from build123d import *

# Parameters (mm, degrees)
F1_DEPTH = 22
F4_DEPTH = 19
F5_R     = 2.5
F6_DEPTH = 5
F7_R     = 4.5
F8_DEPTH = 8


with BuildPart() as f1:
    # F0 (on Top) → F1 (new body)
    with BuildSketch(Plane.XY):
        with BuildLine():
            ThreePointArc((-32.5, 0), (0, 25), (32.5, 0))
            Line((32.5, 0), (49.369318, 0))
            Line((49.369318, 0), (49.369318, 2.5))
            Line((49.369318, 2.5), (34.369318, 2.5))
            ThreePointArc((34.369318, 2.5), (0, 27.5), (-34.369318, 2.5))
            Line((-34.369318, 2.5), (-49.369318, 2.5))
            Line((-49.369318, 2.5), (-49.369318, 0))
            Line((-49.369318, 0), (-32.5, 0))
        make_face()
        with BuildLine():
            Line((49.369318, 0), (32.5, 0))
            ThreePointArc((32.5, 0), (0, -25), (-32.5, 0))
            Line((-32.5, 0), (-49.369318, 0))
            Line((-49.369318, 0), (-49.369318, -2.5))
            Line((-49.369318, -2.5), (-34.369318, -2.5))
            ThreePointArc((-34.369318, -2.5), (0, -27.5), (34.369318, -2.5))
            Line((34.369318, -2.5), (49.369318, -2.5))
            Line((49.369318, -2.5), (49.369318, 0))
        make_face()
    extrude(amount=F1_DEPTH)

    # F3 (on offset) → F4 (join)
    with BuildSketch(Plane.XZ.offset(25)):
        Polygon((6, 11), (2.932883, 16), (-2.932883, 16), (-6, 11), (-2.932883, 6), (2.932883, 6), align=None)
    extrude(amount=F4_DEPTH)

    # F5 (on face) → F6 (cut, through all)
    with BuildSketch(Plane.XZ.offset(2.5)):
        with Locations((41.5, 11)):
            Circle(F5_R)
        with Locations((-41.5, 11)):
            Circle(F5_R)
    extrude(amount=-F6_DEPTH, mode=Mode.SUBTRACT)

    # F7 (on face) → F8 (cut)
    with BuildSketch(Plane.XZ.offset(44)):
        with Locations((0, 11)):
            Circle(F7_R)
    extrude(amount=-F8_DEPTH, mode=Mode.SUBTRACT)


solid = f1.part
Geometry check sheet. Reference: the model listing, model coordinates, mm. A direction names the side the tool comes from. Round coordinates to 2 decimals unless told otherwise and drop trailing zeros. Order: outer loops, then holes, each group sorted by start corner. A loop starts at its lowest first (then second) coordinate and runs counter-clockwise, first axis right, second up. Notation, with made-up numbers: M 83,86.25 L 137,86.25 A18 ccw 137,94.25 Z; hole C -20.75,65 d9. An arc over 180 degrees is marked long. Answer in a Markdown table with one row per item. Add a question column.
Item 1: Draft check along X on faces 5 (the face through (49.369, 0, 11)), 6 (the face through (0, -36, 11)), 7 (the face through (-49.369, 0, 11)). Enter one of: released by +X, released by -X, zero draft, split by the parting line, or undercut.
Item 2: Sectioned sample at A-A, the plane x = 0. Enter the section's corners in (y, z), plus the area to 3 significant figures.
Item 3: Material ranges on L1, parallel to Z at x = 0, y = -39.75; L2, parallel to Z at x = 41.5, y = 0.05; L3, parallel to Y at x = 44.5, z = 16, recorded low to high. Write a range as [from, to].
Item 4: Sectioned sample at D-D, the plane x = -41.5. Enter the section's corners in (y, z).
Item 5: Sectioned sample at B-B, the plane z = 19.25. Enter the section's corners in (x, y) (3 decimals).
Item 6: Sectioned sample at C-C, the plane y = 3.5. Enter the section's corners in (x, z), plus the area to 3 significant figures.
Item 7: Set-up check for faces 1 (the face through (42, 2.5, 8)), 2 (the face through (4.49, -35.38, 13.46)), 3 (the face through (4.44, -35.38, 8.46)), 4 (the face through (-42, -2.5, 8)): record each of +Z, -Z, +X, -X, +Y, -Y from which the full face is reachable in a straight line by a thin tool's end or side.
Item 8: Depth check by flat-ended pin: pin 1 Ø8 at (y, z) = (-27.5, 11) entering from +X; pin 2 Ø4 at (y, z) = (-18, 5) entering from +X; pin 3 Ø12 at (y, z) = (10.5, 8) entering from +X; pin 4 Ø10 at (x, y) = (-12, 12) entering from +Z. Enter the tip coordinate at first touch or a pass-through.
Filled in:
| question | item | result |
|---|---|---|
| 1 | face 5 | released by +X |
| 1 | face 6 | undercut |
| 1 | face 7 | released by -X |
| 2 | outline | M -44,6 L -27.5,6 L -27.5,0 L -25,0 L -25,22 L -27.5,22 L -27.5,16 L -44,16 L -44,15.5 L -36,15.5 L -36,6.5 L -44,6.5 Z; M 25,0 L 27.5,0 L 27.5,22 L 25,22 Z |
| 2 | area | 203 mm² |
| 3 | L1 | z = [6, 6.5], [15.5, 16] |
| 3 | L2 | z = [0, 8.5], [13.5, 22] |
| 3 | L3 | y = [-2.5, 2.5] |
| 4 | outline | M -2.5,0 L 2.5,0 L 2.5,8.5 L -2.5,8.5 Z; M -2.5,13.5 L 2.5,13.5 L 2.5,22 L -2.5,22 Z |
| 5 | outline | M -49.369,-2.5 L -34.369,-2.5 A36.125 ccw 34.369,-2.5 L 49.369,-2.5 L 49.369,2.5 L 34.369,2.5 A36.125 ccw -34.369,2.5 L -49.369,2.5 Z; hole M -32.5,0 A33.625 ccw 32.5,0 A33.625 ccw Z |
| 6 | outline | M -34.03,0 L -31.36,0 L -31.36,22 L -34.03,22 Z; M 31.36,0 L 34.03,0 L 34.03,22 L 31.36,22 Z |
| 6 | area | 117 mm² |
| 7 | face 1 | +Z, -Z, +X, +Y |
| 7 | face 2 | +Z, +X, -Y |
| 7 | face 3 | -Z, +X, -Y |
| 7 | face 4 | +Z, -Z, -X, -Y |
| 8 | pin 1 | stops at x = 16.52 |
| 8 | pin 2 | stops at x = 26.43 |
| 8 | pin 3 | stops at x = 33.66 |
| 8 | pin 4 | passes through |
